Verification items for the finished model (mm, model axes). A direction names the side the tool comes from. Coordinates: 2 decimals unless noted, no trailing zeros. Order: outer loops, then holes, each group sorted by start corner. A loop starts at its lowest first (then second) coordinate and runs counter-clockwise, first axis right, second up. Notation, with made-up numbers: M 24,-4.75 L 67,-4.75 A30 cw 67,22.25 Z; hole C 52.25,1.5 d10. An arc over 180 degrees is marked long. Return JSON: item names as keys, results as strings. Group by question number.
Q1. Thickness scan on probe 1 along Z at (x, y) = (0, -16.7); probe 2 along Z at (x, y) = (12.5, -12); probe 3 along Z at (x, y) = (-12.5, -1.2). Record the ranges inside material, lowest first.
Q2. Section check A-A, the plane x = -12.5. Enter the section's corners in (y, z), then the cut area to 3 significant figures.
Q3. Section check C-C, the plane y = -9.75. Enter the section's corners in (x, z).
Q4. Section check B-B, the plane z = 12.5. Enter the section's corners in (x, y), then the cut area to 3 significant figures.
Q5. Access from +Z, -Z, +X, -X, +Y, -Y to the whole of each face (thin tool, end or side, straight path). Record for faces 4 (the face through (6.4, -19, 4)), 5 (the face through (0, -9, 15.5)), 6 (the face through (0, -20, -4)), 7 (the face through (-12, 0, -8)), 8 (the face through (14, -1.5, 14)).
Q6. Go/stop test with flat-tipped pins: pin 1 Ø6 at (x, z) = (0, -12.04) entering from -Y; pin 2 Ø4.5 at (x, z) = (0, -12.04) entering from -Y; pin 3 Ø3 at (x, y) = (0, -4) entering from +Z; pin 4 Ø2 at (x, z) = (13.5, 13) entering from -Y. Record where each tip stops, or that it passes through.
Q7. Section check D-D, the plane z = 4.5. Enter the section's corners in (x, y), then the cut area to 3 significant figures.
Q8. Mould release check, pull along Z, two halves, no side actions. Record for faces 1 (the face through (0, -10, 17.5)), 2 (the face through (-17.5, -10, 0)), 3 (the face through (-15.747, -10.62, -12.643)): pulls with the +Z half, pulls with the -Z half, needs draft (parallel to the pull), parting line crosses it, or undercut.
from build123d import *

# Parameters (mm, degrees)
SKETCH2_W           = 35
SKETCH2_H           = 35
BOSS_EXTRUDE1_DEPTH = 20
CUT_EXTRUDE1_START  = -1.5
SKETCH4_R           = 3.25
CUT_EXTRUDE1_DEPTH  = 19.5
CAVITY_DEPTH        = 18
SKETCH10_R          = 3.5
SKETCH10_R_2        = 2.6
BOSS_EXTRUDE4_DEPTH = 2
SKETCH8_R           = 1.75
M3_HOLES_DEPTH      = 21
SKETCH9_R           = 2.6
HOLESS_DEPTH        = 3
CUT_EXTRUDE8_REACH  = 37
SKETCH12_R          = 2


with BuildPart() as part:
    # Sketch2 → Boss-Extrude1 (new body)
    with BuildSketch(Plane(origin=(0, 0, 0), x_dir=(1, 0, 0), z_dir=(0, 1, 0))):
        Rectangle(SKETCH2_W, SKETCH2_H)
    extrude(amount=-BOSS_EXTRUDE1_DEPTH)

    # Sketch4 → Cut-Extrude1 (cut, through all)
    with BuildSketch(Plane(origin=(0, 0, 0), x_dir=(1, 0, 0), z_dir=(0, 1, 0)).offset(CUT_EXTRUDE1_START)):
        with Locations((-12.5, 12.5)):
            Circle(SKETCH4_R)
        with Locations((12.5, 12.5)):
            Circle(SKETCH4_R)
        with Locations((-12.5, -12.5)):
            Circle(SKETCH4_R)
        with Locations((12.5, -12.5)):
            Circle(SKETCH4_R)
    extrude(amount=-CUT_EXTRUDE1_DEPTH, mode=Mode.SUBTRACT)

    # Sketch5 → cavity (cut)
    with BuildSketch(Plane(origin=(0, 0, 0), x_dir=(1, 0, 0), z_dir=(0, 1, 0))):
        with BuildLine():
            Line((-8.191578015, 15.5), (0, 15.5))
            Line((0, 15.5), (8.191578015, 15.5))
            ThreePointArc((8.191578015, 15.5), (8.787689399, 8.787689399), (15.5, 8.191578015))
            Line((15.5, 8.191578015), (15.5, 0))
            Line((15.5, 0), (15.5, -8.191578015))
            ThreePointArc((15.5, -8.191578015), (8.787689399, -8.787689399), (8.191578015, -15.5))
            Line((8.191578015, -15.5), (0, -15.5))
            Line((0, -15.5), (-8.191578015, -15.5))
            ThreePointArc((-8.191578015, -15.5), (-8.787689399, -8.787689399), (-15.5, -8.191578015))
            Line((-15.5, -8.191578015), (-15.5, 0))
            Line((-15.5, 0), (-15.5, 8.191578015))
            ThreePointArc((-15.5, 8.191578015), (-8.787689399, 8.787689399), (-8.191578015, 15.5))
        make_face()
    extrude(amount=-CAVITY_DEPTH, mode=Mode.SUBTRACT)

    # Sketch10 → Boss-Extrude4 (add)
    with BuildSketch(Plane(origin=(0, -18, 0), x_dir=(1, 0, 0), z_dir=(0, 1, 0))):
        with Locations((0, 12.040793939)):
            Circle(SKETCH10_R)
        with Locations((0, 12.040793939)):
            Circle(SKETCH10_R_2, mode=Mode.SUBTRACT)
    extrude(amount=BOSS_EXTRUDE4_DEPTH)

    # Sketch8 (on Top Plane) → M3 holes (cut, through all)
    with BuildSketch(Plane(origin=(0, 0, 0), x_dir=(1, 0, 0), z_dir=(0, 1, 0))):
        with Locations((-12.5, 12.5)):
            Circle(SKETCH8_R)
        with Locations((12.5, 12.5)):
            Circle(SKETCH8_R)
        with Locations((12.5, -12.5)):
            Circle(SKETCH8_R)
        with Locations((-12.5, -12.5)):
            Circle(SKETCH8_R)
    extrude(amount=-M3_HOLES_DEPTH, mode=Mode.SUBTRACT)

    # Sketch9 → holess (cut, through all)
    with BuildSketch(Plane(origin=(0, -18, 0), x_dir=(1, 0, 0), z_dir=(0, 1, 0))):
        with Locations((0, 12.040793939)):
            Circle(SKETCH9_R)
        with BuildLine():
            Line((6.4, -1.921240608), (6.4, -7.078759392))
            ThreePointArc((6.4, -7.078759392), (-6.9, -4.5), (6.4, -1.921240608))
        make_face()
    extrude(amount=-HOLESS_DEPTH, mode=Mode.SUBTRACT)

    # Sketch12 → Cut-Extrude8 (cut, up to next)
    with BuildSketch(Plane.XY.offset(17.5), mode=Mode.PRIVATE) as cut_extrude8_sk1:
        with Locations((0, -4)):
            Circle(SKETCH12_R)
    cut_extrude8_tool1 = extrude(cut_extrude8_sk1.sketch, amount=-CUT_EXTRUDE8_REACH, mode=Mode.PRIVATE) & part.part
    add(cut_extrude8_tool1.solids().sort_by_distance((0, -4, 17.5))[0], mode=Mode.SUBTRACT)


solid = part.part
Numbers:
{
 "1": {"probe 1": "z = -17.5 to -14.64, -9.44 to -8.54, 15.5 to 17.5", "probe 2": "z = -17.5 to -15.75, -9.25 to -7.25, 7.25 to 9.25, 15.75 to 17.5", "probe 3": "z = -17.5 to -14.25, -10.75 to -7.25, 7.25 to 10.75, 14.25 to 17.5"},
 "2": {"outline": "M -20,-17.5 L 0,-17.5 L 0,-14.25 L -1.5,-14.25 L -1.5,-15.75 L -20,-15.75 Z; M -20,-9.25 L -1.5,-9.25 L -1.5,-10.75 L 0,-10.75 L 0,-7.25 L -18,-7.25 L -18,7.25 L 0,7.25 L 0,10.75 L -1.5,10.75 L -1.5,9.25 L -20,9.25 Z; M -20,15.75 L -1.5,15.75 L -1.5,14.25 L 0,14.25 L 0,17.5 L -20,17.5 Z", "area": "188 mm2"},
 "3": {"outline": "M -17.5,-17.5 L 17.5,-17.5 L 17.5,17.5 L -17.5,17.5 Z; hole C -12.5,-12.5 d6.5; hole C -12.5,12.5 d6.5; hole M -15.5,-8.19 A5.25 cw -8.19,-15.5 L 8.19,-15.5 A5.25 cw 15.5,-8.19 L 15.5,8.19 A5.25 cw 8.19,15.5 L -8.19,15.5 A5.25 cw -15.5,8.19 Z; hole C 12.5,-12.5 d6.5; hole C 12.5,12.5 d6.5"},
 "4": {"outline": "M -17.5,-20 L -15.75,-20 L -15.75,-1.5 L -14.25,-1.5 L -14.25,0 L -17.5,0 Z; M -10.75,-1.5 L -9.25,-1.5 L -9.25,-20 L 9.25,-20 L 9.25,-1.5 L 10.75,-1.5 L 10.75,0 L 7.25,0 L 7.25,-18 L -7.25,-18 L -7.25,0 L -10.75,0 Z; M 14.25,-1.5 L 15.75,-1.5 L 15.75,-20 L 17.5,-20 L 17.5,0 L 14.25,0 Z", "area": "188 mm2"},
 "5": {"face 4": "+Y, -Y", "face 5": "+Y", "face 6": "+Z, -Z, +X, -X, -Y", "face 7": "+Z, -Z, +X, -X, +Y", "face 8": "-Y"},
 "6": {"pin 1": "stops at y = -20", "pin 2": "passes through", "pin 3": "stops at z = -15.5", "pin 4": "stops at y = -1.5"},
 "7": {"outline": "M -17.5,-20 L -6.9,-20 L -6.9,-18 L -15.5,-18 L -15.5,0 L -17.5,0 Z; M 6.4,-20 L 17.5,-20 L 17.5,0 L 15.5,0 L 15.5,-18 L 6.4,-18 Z", "area": "115 mm2"},
 "8": {"face 1": "pulls with the +Z half", "face 2": "needs draft", "face 3": "undercut"}
}
